```python
from build123d import *

# Parameters (mm, degrees)
SKETCH3_R               = 9
BOSS_EXTRUDE1_DEPTH     = 4
CHAMFER1_SIZE           = 5.196152423
CHAMFER1_SIZE_2         = 3
CUT_EXTRUDE2_DEPTH      = 27.561249971
CUT_EXTRUDE2_DEPTH_BACK = 27.561249971
FILLET1_R               = 0.4
SKETCH6_W               = 1.050125629
SKETCH6_H               = 2
BOSS_EXTRUDE2_DEPTH     = 3
SKETCH7_W               = 6
SKETCH7_H               = 1.5
BOSS_EXTRUDE3_DEPTH     = 8
CHAMFER2_SIZE           = 1


with BuildPart() as part:
    # Sketch2 → Revolve1 (revolve)
    with BuildSketch(Plane(origin=(0, 0, 0), x_dir=(0, 0, -1), z_dir=(1, 0, 0))):
        Polygon((0, 0), (0, 17), (10.5, 17), (11.5, 16), (11.5, 15), (10, 15), (10, 0), align=None)
    revolve(axis=Axis((0, 0, 0), (0, 1, 0)))

    # Sketch3 → Boss-Extrude1 (add)
    with BuildSketch(Plane(origin=(0, 17, 0), x_dir=(1, 0, 0), z_dir=(0, 1, 0))):
        with Locations(Location((0, 0, 0), (0, 0, 270))):
            Circle(SKETCH3_R)
    extrude(amount=BOSS_EXTRUDE1_DEPTH)

    # Chamfer1
    # the kernel refuses this chamfer: 5.196152423, 3 mm, written as the material it takes off along each edge
    with BuildSketch(Plane(origin=(0, 21, 0), x_dir=(0, 0, 1), z_dir=(-1, 0, 0))) as chamfer1_piece_1_section:
        Polygon((9, -CHAMFER1_SIZE), (9 - CHAMFER1_SIZE_2, 0), (9, 0), align=None)
    chamfer1_piece_1 = revolve(axis=Axis((0, 21, 0), (0, 1, 0)), mode=Mode.PRIVATE)
    chamfer1_piece_1 = split(chamfer1_piece_1, bisect_by=Plane(origin=(0, 17, -7.167132971), z_dir=(0, 1, 0)), keep=Keep.TOP, mode=Mode.PRIVATE)
    add(chamfer1_piece_1, mode=Mode.SUBTRACT)

    # Sketch5 → Cut-Extrude2 (cut, two sides: drawn at the far end of the back side and taken through both)
    with BuildSketch(Plane(origin=(0, 0, 0), x_dir=(0, 0, -1), z_dir=(1, 0, 0)).offset(-CUT_EXTRUDE2_DEPTH_BACK)):
        with BuildLine():
            Line((6, 21), (-6, 21))
            Line((-6, 21), (-8.085535149, 17.44220036))
            ThreePointArc((-8.085535149, 17.44220036), (-0.821567104, 18.345354686), (6, 21))
        make_face()
    extrude(amount=CUT_EXTRUDE2_DEPTH + CUT_EXTRUDE2_DEPTH_BACK, mode=Mode.SUBTRACT)

    # Fillet1
    fillet1_edges = [part.edges().sort_by_distance(p)[0] for p in [
        (-9.3e-08, 21, -6),
    ]]
    fillet(fillet1_edges, radius=FILLET1_R)

    # Sketch6 → Boss-Extrude2 (add)
    with BuildSketch(Plane.XZ.offset(-15)):
        with Locations((-10.474937185, 0)):
            Rectangle(SKETCH6_W, SKETCH6_H)
    extrude(amount=BOSS_EXTRUDE2_DEPTH)

    # Sketch7 → Boss-Extrude3 (add)
    with BuildSketch(Plane.XZ):
        Rectangle(SKETCH7_W, SKETCH7_H)
        with Locations((0, 7.25)):
            Rectangle(SKETCH7_W, SKETCH7_H)
    extrude(amount=BOSS_EXTRUDE3_DEPTH)

    # Chamfer2
    chamfer2_edges = [part.edges().sort_by_distance(p)[0] for p in [
        (0, 0, 10),
    ]]
    chamfer(chamfer2_edges, length=CHAMFER2_SIZE)


solid = part.part
```
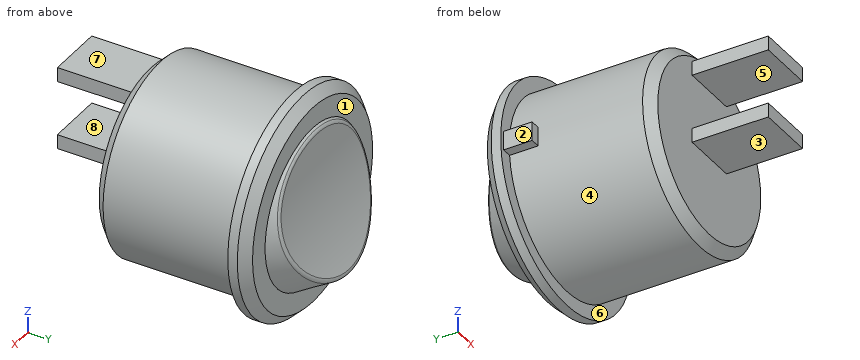
Geometry check sheet. Reference: the model listing, model coordinates, mm. Face numbers are marked on the shaded views. A direction names the side the tool comes from. Round coordinates to 2 decimals unless told otherwise and drop trailing zeros. Order: outer loops, then holes, each group sorted by start corner. A loop starts at its lowest first (then second) coordinate and runs counter-clockwise, first axis right, second up. Notation, with made-up numbers: (24, -7.75) -> (45, -7.75) arc R31 ccw to (45, 21.25) -> close; hole circle Ø8 at (-7.5, -37.75). An arc over 180 degrees is marked (long way). Return JSON: item names as keys, results as strings. Group by question number.
Q1. Section check C-C, the plane y = 13.5. Record the boundary of the cut face in (x, z), plus the area to 3 significant figures.
Q2. Section check B-B, the plane y = 5. Record the boundary of the cut face in (x, z).
Q3. Release check for a two-part mould opening along Z. For the marked faces 6, 7 and 8 record: released by +Z, released by -Z, zero draft, split by the parting line, or undercut.
Q4. Section check A-A, the plane y = -3.25. Record the boundary of the cut face in (x, z).
Q5. Tool access check on the marked faces 1, 2, 3, 4 and 5. Record the directions out of +Z, -Z, +X, -X, +Y, -Y that give a thin tool (end or side, any length) a straight path to the whole face; none if there is none.
Q6. Material ranges on probe 1 along Z at (x, y) = (2.5, -3.75); probe 2 along Y at (x, z) = (-8.5, -0.25); probe 3 along X at (y, z) = (13, 0.25), recorded low to high. Write a range as from..to.
Q7. Gauge pin test, flat ends, axial feed: pin 1 (1.6 mm diameter, centred on y = -2, z = -0.5, fed in from +X); pin 2 (1.5 mm diameter, centred on x = -3.5, z = 0.5, fed in from +Y); pin 3 (2 mm diameter, centred on y = 13, z = 0, fed in from -X). Record the tip position at first contact, or that the pin passes through.
Numbers:
{
 "1": {"outline": "(-11, -1) -> (-9.95, -1) arc R10 ccw (long way) to (-9.95, 1) -> (-11, 1) -> close", "area": "316 mm^2"},
 "2": {"outline": "circle Ø20 at (0, 0)"},
 "3": {"face 6": "zero draft", "face 7": "released by +Z", "face 8": "undercut"},
 "4": {"outline": "(-3, -0.75) -> (3, -0.75) -> (3, 0.75) -> (-3, 0.75) -> close; (-3, 6.5) -> (3, 6.5) -> (3, 8) -> (-3, 8) -> close"},
 "5": {"face 1": "+Y", "face 2": "+Z, -Z, -X, -Y", "face 3": "-Z, +X, -X, -Y", "face 4": "-Y", "face 5": "+X, -X, -Y"},
 "6": {"probe 1": "-0.75..0.75, 6.5..8", "probe 2": "0..17", "probe 3": "-11..10"},
 "7": {"pin 1": "x = 3", "pin 2": "y = 18.64", "pin 3": "x = -11"}
}
